Design review of the part built by this model. Coordinates are the model's own, in mm. A direction names the side the tool comes from. Give positions to 0.01 mm unless a question says otherwise; leave off trailing zeros. Write each loop counter-clockwise with the first axis right and the second up, starting at its lowest first coordinate (ties: lowest second). Pieces come first, ordered by that corner, then holes. Notation, with made-up numbers: (12, 42) -> (23, 42) arc R22 cw to (23, 57) -> close; hole circle Ø5 at (43.25, 49.5). An arc over 180 degrees is marked (long way). Answer as a JSON object with one key per item and string values.
```python
from build123d import *

# Parameters (mm, degrees)
BOSS_EXTRUDE1_DEPTH = 20
SKETCH2_R           = 1.7
CUT_EXTRUDE1_DEPTH  = 28.75
CUT_EXTRUDE2_REACH  = 61.184
SKETCH4_R           = 2.25
CHAMFER1_SIZE       = 1
CUT_EXTRUDE3_REACH  = 155.199
SKETCH5_R           = 3.3


with BuildPart() as part:
    # Sketch1 → Boss-Extrude1 (new body)
    with BuildSketch(Plane(origin=(0, 0, 0), x_dir=(1, 0, 0), z_dir=(0, 1, 0))):
        with BuildLine():
            Line((23.75, 120.769174208), (23.75, 134.895099729))
            Line((23.75, 134.895099729), (21.25, 134.895099729))
            Line((21.25, 134.895099729), (21.25, 123.995190528))
            ThreePointArc((21.25, 123.995190528), (17.839743095, 119.73175291), (18.223690728, 114.285714286))
            ThreePointArc((18.223690728, 114.285714286), (18.048629784, 111.396432549), (15.513167019, 110))
            Line((15.513167019, 110), (-15.513167019, 110))
            ThreePointArc((-15.513167019, 110), (-18.048629784, 111.396432549), (-18.223690728, 114.285714286))
            ThreePointArc((-18.223690728, 114.285714286), (-17.839743095, 119.73175291), (-21.25, 123.995190528))
            Line((-21.25, 123.995190528), (-21.25, 134.895099729))
            Line((-21.25, 134.895099729), (-23.75, 134.895099729))
            Line((-23.75, 134.895099729), (-23.75, 120.769174208))
            ThreePointArc((-23.75, 120.769174208), (-25, 114), (-26.25, 120.769174208))
            Line((-26.25, 120.769174208), (-26.25, 134.895099729))
            Line((-26.25, 134.895099729), (-28.75, 134.895099729))
            Line((-28.75, 134.895099729), (-28.75, 123.995190528))
            ThreePointArc((-28.75, 123.995190528), (-31.495190528, 121.25), (-32.5, 117.5))
            Line((-32.5, 117.5), (-37.5, 117.5))
            Line((-37.5, 117.5), (-42.5, 108.839745962))
            Line((-42.5, 108.839745962), (-37.000738686, 105.664745962))
            Line((-37.000738686, 105.664745962), (-47.000738686, 88.344237886))
            Line((-47.000738686, 88.344237886), (-42.670611667, 85.844237886))
            Line((-42.670611667, 85.844237886), (-31.611027254, 105))
            Line((-31.611027254, 105), (31.611027254, 105))
            Line((31.611027254, 105), (42.670611667, 85.844237886))
            Line((42.670611667, 85.844237886), (47.000738686, 88.344237886))
            Line((47.000738686, 88.344237886), (37.000738686, 105.664745962))
            Line((37.000738686, 105.664745962), (42.5, 108.839745962))
            Line((42.5, 108.839745962), (37.5, 117.5))
            Line((37.5, 117.5), (32.5, 117.5))
            ThreePointArc((32.5, 117.5), (31.495190528, 121.25), (28.75, 123.995190528))
            Line((28.75, 123.995190528), (28.75, 134.895099729))
            Line((28.75, 134.895099729), (26.25, 134.895099729))
            Line((26.25, 134.895099729), (26.25, 120.769174208))
            ThreePointArc((26.25, 120.769174208), (25, 114), (23.75, 120.769174208))
        make_face()
    extrude(amount=BOSS_EXTRUDE1_DEPTH)

    # Sketch2 → Cut-Extrude1 (cut, symmetric)
    with BuildSketch(Plane(origin=(0, 0, 0), x_dir=(0, 0, -1), z_dir=(1, 0, 0))):
        with Locations((129.445145129, 10)):
            Circle(SKETCH2_R)
    extrude(amount=CUT_EXTRUDE1_DEPTH, both=True, mode=Mode.SUBTRACT)

    # Sketch4 → Cut-Extrude2 (cut, up to next)
    with BuildSketch(Plane.XY.offset(-105), mode=Mode.PRIVATE) as cut_extrude2_sk1:
        with Locations((0, 15)):
            Circle(SKETCH4_R)
    cut_extrude2_tool1 = extrude(cut_extrude2_sk1.sketch, amount=-CUT_EXTRUDE2_REACH, mode=Mode.PRIVATE) & part.part
    add(cut_extrude2_tool1.solids().sort_by_distance((0, 15, -105))[0], mode=Mode.SUBTRACT)

    # Chamfer1
    chamfer1_edges = [part.edges().sort_by_distance(p)[0] for p in [
        (25, 20, -114),
        (-25, 20, -114),
    ]]
    chamfer(chamfer1_edges, length=CHAMFER1_SIZE)

    # Sketch5 → Cut-Extrude3 (cut, up to next)
    with BuildSketch(Plane(origin=(-73.504731158, 0, -42.437976321), x_dir=(-0.49999999999998673, 0, 0.8660254037844464), z_dir=(-0.8660254037844464, 0, -0.49999999999998673)), mode=Mode.PRIVATE) as cut_extrude3_sk1:
        with Locations((-63.007984945, 10)):
            Circle(SKETCH5_R)
    cut_extrude3_tool1 = extrude(cut_extrude3_sk1.sketch, amount=-CUT_EXTRUDE3_REACH, mode=Mode.PRIVATE) & part.part
    cut_extrude3 = cut_extrude3_tool1.solids().sort_by_distance((-42.000739, 10, -97.004492))[0]
    add(cut_extrude3, mode=Mode.SUBTRACT)

    # Mirror1: Cut-Extrude3 across plane
    add(cut_extrude3.mirror(Plane(origin=(0, 0, 0), x_dir=(0, 0, 1), z_dir=(1, 0, 0))), mode=Mode.SUBTRACT)


solid = part.part
```
(1) We need section C-C, the plane z = -102. State the section outline as (x, y) points, then the cut area to 3 significant figures.
Here are the results:
{"outline": "(-39.12, 0) -> (-33.34, 0) -> (-33.34, 20) -> (-39.12, 20) -> close; (33.34, 0) -> (39.12, 0) -> (39.12, 20) -> (33.34, 20) -> close", "area": "231 mm²"}
(2) We need section B-B, the plane z = -129. Give the number of separate pieces and of enclosed holes in the cut face, then the cut area to 3 significant figures.
Here are the results:
{"separate pieces": "8", "enclosed holes": "0", "area": "167 mm²"}
(3) The part is to be moulded in two halves that separate along Y. For faces 1 (the flat face through (26.25, 10, -126)), 2 (the flat face through (0, 20, -107)), 3 (the cylindrical face through (-0.488, 12.804, -107.465)), say which applies: +Y half, -Y half, draft (parallel to the pull), parting line (faces both ways), or undercut.
Here are the results:
{"face 1": "draft", "face 2": "+Y half", "face 3": "undercut"}
(4) For line 1 along X through (y, z) = (3.25, -129); line 2 along Z through (x, y) = (-23, 11.25); line 3 along Y through (x, z) = (0, -106.9), list the stretches that pass through material, from the lowest coordinate up.
Here are the results:
{"line 1": "x = -28.75 to -26.25, -23.75 to -21.25, 21.25 to 23.75, 26.25 to 28.75", "line 2": "z = -134.9 to -130.6, -128.29 to -120.37, -114.63 to -105", "line 3": "y = 0 to 12.75, 17.25 to 20"}
(5) We need section A-A, the plane x = 0. State the section outline as (y, z) points, then the cut area to 3 significant figures.
Here are the results:
{"outline": "(0, -110) -> (12.75, -110) -> (12.75, -105) -> (0, -105) -> close; (17.25, -110) -> (20, -110) -> (20, -105) -> (17.25, -105) -> close", "area": "77.5 mm²"}
(6) Clearance check with flat-ended pins moving along their axes: pin 1 (4 mm diameter, centred on y = 8, z = -129, fed in from +X); pin 2 (5.5 mm diameter, centred on y = 8.5, z = -130.5, fed in from -X); pin 3 (7 mm diameter, centred on x = 0, y = 15, fed in from +Z); pin 4 (2 mm diameter, centred on y = 10, z = -129.45, fed in from +X). State where each tip first meets the part, or that it passes through.
Here are the results:
{"pin 1": "stops at x = 28.75", "pin 2": "stops at x = -28.75", "pin 3": "stops at z = -105", "pin 4": "passes through"}
(7) For faces 4 (the flat face through (0, 10, -105)), 5 (the flat face through (28.75, 8, -129)), 6 (the cylindrical face through (-17.817, 9.86, -119.657)), 7 (the flat face through (39.71, 9.86, -107.23)), 8 (the flat face through (-21.25, 8, -129)), list the 3-axis set-ups (+Z, -Z, +X, -X, +Y, -Y) from which the entire face can be reached by the end or side of a thin tool; tool diameter is ignored.
Here are the results:
{"face 4": "+Z, +Y, -Y", "face 5": "-Z, +X, +Y, -Y", "face 6": "+Y, -Y", "face 7": "+X, +Y, -Y", "face 8": "-Z, +Y, -Y"}
(8) We need section D-D, the plane x = -25. State the section outline as (y, z) points, then the cut area to 4 significant figures.
Here are the results:
{"outline": "(0, -114) -> (19, -114) -> (20, -113) -> (20, -105) -> (0, -105) -> close", "area": "179.5 mm²"}
